from build123d import *

# Parameters (mm, degrees)
SKETCH_1_W          = 70
SKETCH_1_H          = 60
EXTRUDE_1_DEPTH     = 12
CUT_EXTRUDE_1_REACH = 49.634
SKETCH_2_R          = 18


with BuildPart() as part:
    # 草图1 → 凸台-拉伸1 (new body)
    with BuildSketch(Plane.XY):
        Rectangle(SKETCH_1_W, SKETCH_1_H)
    extrude(amount=EXTRUDE_1_DEPTH)

    # 草图2 → 切除-拉伸1 (cut, up to next)
    with BuildSketch(Plane(origin=(0, 0, 0), x_dir=(-1, 0, 0), z_dir=(0, 0, -1)), mode=Mode.PRIVATE) as cut_extrude_1_sk1:
        Circle(SKETCH_2_R)
    cut_extrude_1_tool1 = extrude(cut_extrude_1_sk1.sketch, amount=-CUT_EXTRUDE_1_REACH, mode=Mode.PRIVATE) & part.part
    add(cut_extrude_1_tool1.solids().sort_by_distance((0, 0, 0))[0], mode=Mode.SUBTRACT)


solid = part.part
Source: CAD feature listing. Evaluate the final solid. Frame: model axes, mm. Round coordinates to 2 decimals unless told otherwise and drop trailing zeros. Order: outer loops, then holes, each group sorted by start corner. A loop starts at its lowest first (then second) coordinate and runs counter-clockwise, first axis right, second up. Notation, with made-up numbers: (38, -21.5) -> (97, -21.5) arc R29 ccw to (97, 13.5) -> close; hole circle Ø10 at (-12.75, -25). An arc over 180 degrees is marked (long way). Answer as CSV lines item,"result".
Item 1: Pin query (flat end, axial travel): pin 1 Ø8 at (x, y) = (21, 13.5) entering from -Z. Return the tip coordinate at first contact, or that it passes through.
A:
pin 1,"z = 0"
Item 2: Line query: L1, parallel to Y at x = 0, z = 3; L2, parallel to X at y = 5.5, z = 5; L3, parallel to X at y = 5, z = 9. Output: solid intervals per line, ascending.
A:
L1,"-30 to -18, 18 to 30"
L2,"-35 to -17.14, 17.14 to 35"
L3,"-35 to -17.29, 17.29 to 35"
Item 3: Section A-A, the plane x = 0. Return loops of the section in (y, z).
A:
outline,"(-30, 0) -> (-18, 0) -> (-18, 12) -> (-30, 12) -> close; (18, 0) -> (30, 0) -> (30, 12) -> (18, 12) -> close"
Item 4: Pull-direction query (X, two-part tool) for faces 1 (the face through (0, 30, 6)), 2 (the face through (2.343, 17.847, 5.916)), 3 (the face through (-35, 0, 6)), 4 (the face through (35, 0, 6)); classes: pulls with the +X half, pulls with the -X half, needs draft (parallel to the pull), parting line crosses it, or undercut.
A:
face 1,"needs draft"
face 2,"undercut"
face 3,"pulls with the -X half"
face 4,"pulls with the +X half"
Item 5: Section C-C, the plane z = 2.5. Return loops of the section in (x, y).
A:
outline,"(-35, -30) -> (35, -30) -> (35, 30) -> (-35, 30) -> close; hole circle Ø36 at (0, 0)"
Item 6: Section B-B, the plane y = 0. Return loops of the section in (x, z).
A:
outline,"(-35, 0) -> (-18, 0) -> (-18, 12) -> (-35, 12) -> close; (18, 0) -> (35, 0) -> (35, 12) -> (18, 12) -> close"
